Source: three-view drawing plus pictorial views. Frame: mm from the lowest corner of the part. Round coordinates to 2 decimals unless told otherwise and drop trailing zeros. Order: outer loops, then holes, each group sorted by start corner. A loop starts at its lowest first (then second) coordinate and runs counter-clockwise, first axis right, second up. Notation, with made-up numbers: (38, 36) - (92, 36) arc R24 ccw to (92, 68) - close; hole circle Ø5 at (67.25, 82). An arc over 180 degrees is marked (long way). Use one line per item in the form item = value. Start each with the question number.
Q1. Cut plane C-C, the plane x = 93. Return the cut outline in (y, z), and give its area (3 significant figures).
Q2. Ray query, line 1 (Y direction, x = 110, z = 0.7); line 2 (Y direction, x = 110, z = 1.7) (3 decimals); line 3 (X direction, y = 7.75, z = 1.95). Return the intervals inside material, ascending. Write a range as [from, to].
Q3. Cut plane A-A, the plane x = 60. Return the cut outline in (y, z).
Q4. Cut plane B-B, the plane z = 1.5. Give the number of separate pieces and of enclosed holes in the cut face, and give its area (3 significant figures).
Q5. Pin query (flat end, axial travel): pin 1 Ø5.5 at (x, y) = (108, 11) entering from +Z. Return the tip coordinate at first contact, or that it passes through.
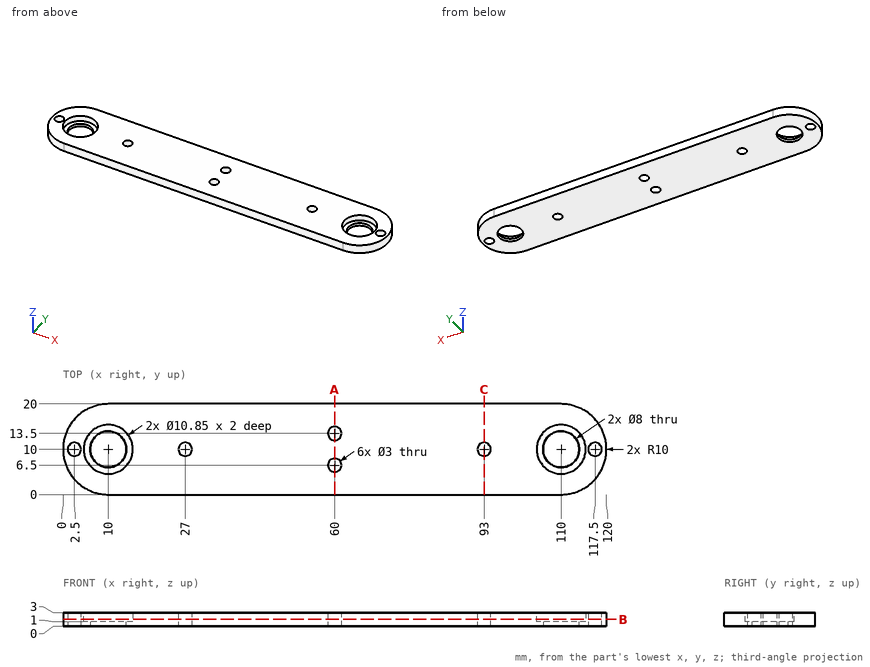
Completed:
q1.outline = (0, 0) - (8.5, 0) - (8.5, 3) - (0, 3) - close; (11.5, 0) - (20, 0) - (20, 3) - (11.5, 3) - close
q1.area = 51.0 mm2
q2.line_1 = [0, 6], [14, 20]
q2.line_2 = [0, 4.575], [15.425, 20]
q2.line_3 = [0.26, 5.06], [14.94, 59.17], [60.83, 105.06], [114.94, 119.74]
q3.outline = (0, 0) - (5, 0) - (5, 3) - (0, 3) - close; (8, 0) - (12, 0) - (12, 3) - (8, 3) - close; (15, 0) - (20, 0) - (20, 3) - (15, 3) - close
q4.separate_pieces = 1
q4.enclosed_holes = 8
q4.area = 2,090 mm2
q5.pin_1 = 1
